Check sheet for the modelled part. Datum: model origin and axes. Units: mm. Face numbers are marked on the shaded views. Give positions to 0.01 mm unless a question says otherwise; leave off trailing zeros. Loops run counter-clockwise (first coordinate to the right, second up) from the corner with the lowest first, then second, coordinate; pieces in that order, holes last. Notation, with made-up numbers: (-7.75, 8.25) -> (41.25, 8.25) arc R12 ccw to (41.25, 23.25) -> close; hole circle Ø10 at (-36, 39.25). An arc over 180 degrees is marked (long way). Answer as CSV lines item,"result". Start each with the question number.
(1) Section check A-A on x = 0. Enter the section's corners in (y, z) (3 decimals).
(2) Section check B-B on z = 5. Enter the section's corners in (x, y) (3 decimals).
(3) Material ranges on line 1 (Y direction, x = 18, z = 2.25); line 2 (Y direction, x = -12.5, z = 6.25); line 3 (X direction, y = -5, z = 1.25), recorded low to high. Write a range as from..to.
(4) Release check for a two-part mould opening along X. For the marked faces 1, 2, 3 and 4 record: pulls with the +X half, pulls with the -X half, needs draft (parallel to the pull), parting line crosses it, or undercut.
(5) Gauge pin test, flat end, axial feed: pin 1 Ø3 at (x, z) = (-9, 4.5) entering from -Y. Record the tip position at first contact, or that the pin passes through.
(6) Section check C-C on y = 0. Enter the section's corners in (x, z) (3 decimals), plus the area to 3 significant figures.
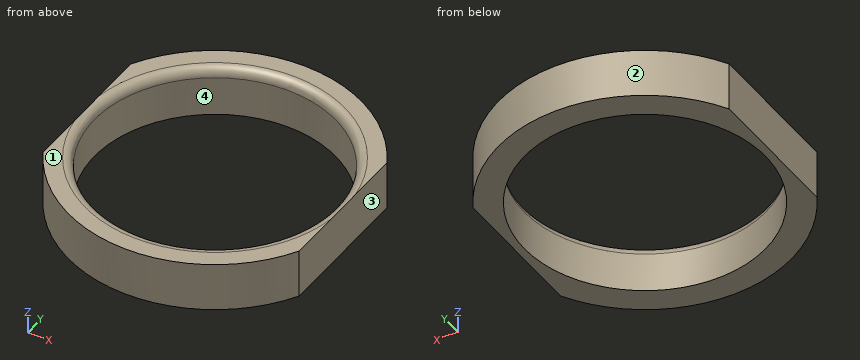
from build123d import *

# Parameters (mm, degrees)
F0_R     = 19.715
F1_DEPTH = 8


# Not quite as in the source:
# - a fillet or chamfer that OpenCascade refuses, or shapes differently, is made with other operations: its cross-section is extruded or revolved along the edge and cut away or added


with BuildPart() as f1:
    # F0 (on Top) → F1 (new body)
    with BuildSketch(Plane.XY):
        with BuildLine():
            Line((20.97, -11.5905435593), (20.97, 11.5905435593))
            ThreePointArc((20.97, 11.5905435593), (0, 23.96), (-20.97, 11.5905435593))
            Line((-20.97, 11.5905435593), (-20.97, -11.5905435593))
            ThreePointArc((-20.97, -11.5905435593), (0, -23.96), (20.97, -11.5905435593))
        make_face()
        Circle(F0_R, mode=Mode.SUBTRACT)
    extrude(amount=F1_DEPTH)

    # F2: fillet of radius 1.5 on 1 edges, made by hand

    # F2_s1 → F2_t2 (revolve, cut)
    with BuildSketch(Plane.XZ):
        with BuildLine():
            ThreePointArc((19.715, 6.5), (20.1543398282, 7.5606601718), (21.215, 8))
            Line((21.215, 8), (19.715, 8))
            Line((19.715, 8), (19.715, 6.5))
        make_face()
    revolve(axis=Axis((0, 0, 8), (0, 0, 1)), mode=Mode.SUBTRACT)


solid = f1.part
Working result:
1,outline,"(-23.96, 0) -> (-19.715, 0) -> (-19.715, 6.5) arc R1.5 ccw to (-21.215, 8) -> (-23.96, 8) -> close; (19.715, 0) -> (23.96, 0) -> (23.96, 8) -> (21.215, 8) arc R1.5 ccw to (19.715, 6.5) -> close"
2,outline,"(-20.97, -11.591) arc R23.96 ccw to (20.97, -11.591) -> (20.97, 11.591) arc R23.96 ccw to (-20.97, 11.591) -> close; hole circle Ø39.43 at (0, 0)"
3,line 1,"y = -15.81..-8.04, 8.04..15.81"
3,line 2,"y = -20.44..-15.25, 15.25..20.44"
3,line 3,"x = -20.97..-19.07, 19.07..20.97"
4,face 1,"needs draft"
4,face 2,"parting line crosses it"
4,face 3,"pulls with the +X half"
4,face 4,"undercut"
5,pin 1,"stops at y = -22.76"
6,outline,"(-20.97, 0) -> (-19.715, 0) -> (-19.715, 6.5) arc R1.5 ccw to (-20.97, 7.98) -> close; (19.715, 0) -> (20.97, 0) -> (20.97, 7.98) arc R1.5 ccw to (19.715, 6.5) -> close"
6,area,"19.1 mm^2"
